```python
from build123d import *

# Parameters (mm, degrees)
F1_W      = 100.959658
F1_H      = 169.9415
F2_DEPTH  = 104.405696
F3_R      = 35.229378
F2_FACE_W = 33.94694
F2_FACE_H = 99.482744
F4_DEPTH  = 65.501096


with BuildPart() as f2:
    # F1 (on face) → F2 (new body)
    with BuildSketch(Plane.XZ):
        with Locations((1.969874, 20.931415)):
            Rectangle(F1_W, F1_H)
    extrude(amount=F2_DEPTH)

    # F3
    f3_edges = [f2.edges().sort_by_distance(p)[0] for p in [
        (52.449703, -52.202848, 105.902165),
        (-48.509955, -52.202848, 105.902165),
        (1.969874, 0, 105.902165),
        (1.969874, -104.405696, 105.902165),
        (52.449703, -52.202848, -64.039335),
        (52.449703, 0, 20.931415),
        (52.449703, -104.405696, 20.931415),
    ]]
    fillet(f3_edges, radius=F3_R)

    # F2_face (on face) → F4 (join)
    with BuildSketch(Plane(origin=(52.449703, -52.202848, 20.931415), x_dir=(0, 1, 0), z_dir=(1, 0, 0))):
        Rectangle(F2_FACE_W, F2_FACE_H)
    extrude(amount=F4_DEPTH)


solid = f2.part
```
Part model, mm, in its own coordinate system. A direction names the side the tool comes from. Coordinates: 2 decimals unless noted, no trailing zeros. Order: outer loops, then holes, each group sorted by start corner. A loop starts at its lowest first (then second) coordinate and runs counter-clockwise, first axis right, second up. Notation, with made-up numbers: (7, 82) - (39, 82) arc R26 ccw to (39, 103) - close; hole circle Ø4 at (44, -38.75). An arc over 180 degrees is marked (long way). Return JSON: item names as keys, results as strings. Group by question number.
Item 1: Cut at B-B (y = -48). List the corners of the cut face in (x, z).
Item 2: Cut at D-D (y = -75). List the corners of the cut face in (x, z), plus the area to 3 significant figures.
Item 3: Which spindle directions (+Z, -Z, +X, -X, +Y, -Y) get a long thin tool onto all of the face, cutting with end or side? Do faces 1 (the face through (85, -52, 70.673)), 2 (the face through (85, -69.176, 20)), 3 (the face through (85, -52, -28.81)), 4 (the face through (85, -35.229, 20)), 5 (the face through (-16, -51, -64.039)). Say none if no direction does.
Item 4: Pin check, flat tips, straight feed: pin 1 (10 mm diameter, centred on x = 83.5, y = -60.5, fed in from +Z); pin 2 (5 mm diameter, centred on x = 50, y = -70, fed in from +Z); pin 3 (19.5 mm diameter, centred on x = 80.5, z = 18, fed in from +Y); pin 4 (12 mm diameter, centred on x = 67, y = -78, fed in from +Z). Stop position of each tip, or through.
Item 5: Cut at C-C (x = 14.5). List the corners of the cut face in (y, z).
Item 6: Cut at A-A (z = -17.5). List the corners of the cut face in (x, y).
Item 7: Drill centre lines: probe 1 along Y at (x, z) = (85.5, -14.5); probe 2 along Z at (x, y) = (89, -65.5); probe 3 along Z at (x, y) = (-13.5, -57.5). Where is each one in solid material? Low to high. Write a range as from..to.
Check values:
{
 "1": {"outline": "(-48.51, -64.04) - (17.22, -64.04) arc R35.23 ccw to (52.45, -28.81) - (117.95, -28.81) - (117.95, 70.67) - (52.45, 70.67) arc R35.23 ccw to (17.22, 105.9) - (-13.28, 105.9) arc R35.23 ccw to (-48.51, 70.67) - close"},
 "2": {"outline": "(-48.51, -64.04) - (17.22, -64.04) arc R35.23 ccw to (51.97, -34.63) - (51.97, 70.67) arc R34.74 ccw to (17.22, 105.42) - (-19.1, 105.42) arc R35.23 ccw to (-48.51, 70.67) - close", "area": "16,300 mm2"},
 "3": {"face 1": "+Z, +X, +Y, -Y", "face 2": "+Z, -Z, +X, -Y", "face 3": "-Z, +X, +Y, -Y", "face 4": "+Z, -Z, +X, +Y", "face 5": "-Z, +X, -X, +Y, -Y"},
 "4": {"pin 1": "stops at z = 70.67", "pin 2": "stops at z = 88.66", "pin 3": "stops at y = -35.23", "pin 4": "passes through"},
 "5": {"outline": "(-104.41, -64.04) - (0, -64.04) - (0, 70.67) arc R35.23 ccw to (-35.23, 105.9) - (-69.18, 105.9) arc R35.23 ccw to (-104.41, 70.67) - close"},
 "6": {"outline": "(-48.51, -104.41) - (17.22, -104.41) arc R35.23 ccw to (52.45, -69.18) - (117.95, -69.18) - (117.95, -35.23) - (52.45, -35.23) arc R35.23 ccw to (17.22, 0) - (-48.51, 0) - close"},
 "7": {"probe 1": "y = -69.18..-35.23", "probe 2": "z = -28.81..70.67", "probe 3": "z = -64.04..105.9"}
}
